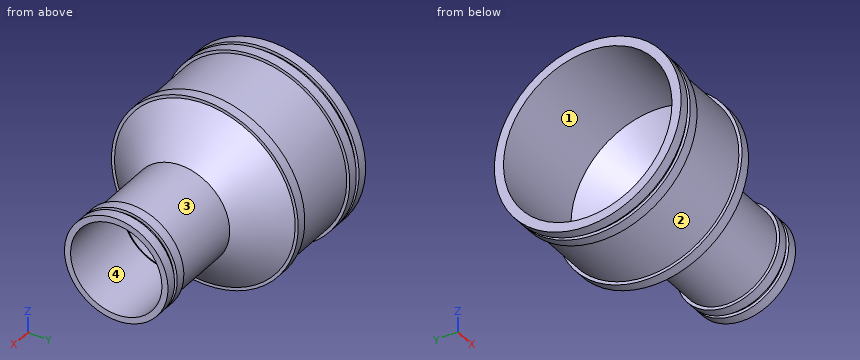
```python
from build123d import *

# Parameters (mm, degrees)
SKELETON_R          = 44.5
SKELETON_R_2        = 41.5
BOSS_EXTRUDE1_DEPTH = 51
BOSS_EXTRUDE2_START = 69
SKELETON_3_R        = 24
SKELETON_3_R_2      = 22
BOSS_EXTRUDE2_DEPTH = 49
SKETCH4_W           = 5
SKETCH4_H           = 1.5
SKETCH6_R           = 22.5
CUT_EXTRUDE1_DEPTH  = 39


with BuildPart() as part:
    # Skeleton → Boss-Extrude1 (new body)
    with BuildSketch(Plane(origin=(0, 0, 0), x_dir=(0, 0, -1), z_dir=(1, 0, 0))):
        Circle(SKELETON_R)
        Circle(SKELETON_R_2, mode=Mode.SUBTRACT)
    extrude(amount=BOSS_EXTRUDE1_DEPTH)



with BuildPart() as body_2:
    # Skeleton<3> → Boss-Extrude2 (new body)
    with BuildSketch(Plane(origin=(0, 0, 0), x_dir=(0, 0, -1), z_dir=(1, 0, 0)).offset(BOSS_EXTRUDE2_START)):
        Circle(SKELETON_3_R)
        Circle(SKELETON_3_R_2, mode=Mode.SUBTRACT)
    extrude(amount=BOSS_EXTRUDE2_DEPTH)


with BuildPart() as part_1:
    add(part.part)

    add(body_2.part)  # loft1 joins it to this body
    # loft up to a face of the part (loft1)
    loft([Face(Wire([part_1.edges().sort_by_distance((51, 32.43910392, 30.462346214))[0]])), Face(Wire([part_1.edges().sort_by_distance((69, -17.495247058, 16.429130542))[0]]))])

    # Cut-Loft1: read off the stored shape, not the designer's step
    # Cut-Loft1: loft between two sections, ruled curve by curve
    cut_loft1_from = [
        Edge.make_bspline([(69, 9.116262782, -20.022331355), (69, -30.928399928, -38.254856919), (69, -49.160925492, 1.789805791), (69, -9.116262782, 20.022331355), (69, 30.928399928, 38.254856919), (69, 49.160925492, -1.789805791), (69, 9.116262782, -20.022331355)], [0, 0, 0, 0, 0.5, 0.5, 0.5, 1, 1, 1, 1], 3, [1, 0.333333333, 0.333333333, 1, 0.333333333, 0.333333333, 1]),
    ]
    cut_loft1_to = [
        Edge.make_bspline([(51, 27.366118575, -31.198486408), (51, -35.030854242, -85.930723557), (51, -89.763091391, -23.533750741), (51, -27.366118575, 31.198486408), (51, 35.030854242, 85.930723557), (51, 89.763091391, 23.533750741), (51, 27.366118575, -31.198486408)], [0, 0, 0, 0, 0.5, 0.5, 0.5, 1, 1, 1, 1], 3, [1, 0.333333333, 0.333333333, 1, 0.333333333, 0.333333333, 1]),
    ]
    cut_loft1 = Solid(Shell([*[Face.make_surface_from_curves(cut_loft1_from[k], cut_loft1_to[k]) for k in range(1)], Face(Wire(cut_loft1_from)), Face(Wire(cut_loft1_to))]))
    add(cut_loft1, mode=Mode.SUBTRACT)

    # Sketch4 → Revolve1 (revolve)
    with BuildSketch(Plane.XY, mode=Mode.PRIVATE) as revolve1_sk:
        with Locations((9.5, 45.25)):
            Rectangle(SKETCH4_W, SKETCH4_H)
        with Locations((2.5, 45.25)):
            Rectangle(SKETCH4_W, SKETCH4_H)
        with Locations((48.5, 45.25)):
            Rectangle(SKETCH4_W, SKETCH4_H)
        with Locations((108.5, 24.75)):
            Rectangle(SKETCH4_W, SKETCH4_H)
        with Locations((115.5, 24.75)):
            Rectangle(SKETCH4_W, SKETCH4_H)
    revolve(revolve1_sk.sketch.rotate(Axis((0, 0, 0), (1, 0, 0)), 90), axis=Axis((0, 0, 0), (1, 0, 0)))

    # Sketch6 → Cut-Extrude1 (cut)
    with BuildSketch(Plane(origin=(118, 0, 0), x_dir=(0, 0, -1), z_dir=(1, 0, 0))):
        Circle(SKETCH6_R)
    extrude(amount=-CUT_EXTRUDE1_DEPTH, mode=Mode.SUBTRACT)


solid = part_1.part
```
Geometry check sheet. Reference: the model listing, model coordinates, mm. Face numbers are marked on the shaded views. A direction names the side the tool comes from. Coordinates: 2 decimals unless noted, no trailing zeros. Loops run counter-clockwise (first coordinate to the right, second up) from the corner with the lowest first, then second, coordinate; pieces in that order, holes last.
Item 1: Sectioned sample at A-A, the plane x = 91. Record the boundary of the cut face in (y, z).
Item 2: Go/stop test with flat-tipped pins: pin 1 Ø8 at (y, z) = (-28.5, 13.5) entering from -X; pin 2 Ø10 at (x, y) = (72.5, -19) entering from -Z; pin 3 Ø10 at (x, y) = (60, -34) entering from +Z; pin 4 Ø10 at (y, z) = (15, -23.5) entering from +X. Record where each tip stops, or that it passes through.
Item 3: Release check for a two-part mould opening along Y. For the marked faces 1 and 2 record: released by +Y, released by -Y, zero draft, split by the parting line, or undercut.
Item 4: Access from +Z, -Z, +X, -X, +Y, -Y to the whole of each face (thin tool, end or side, straight path). Record for the marked faces 3 and 4.
Item 5: Thickness scan on line 1 (X direction, y = 31.5, z = -32.5); line 2 (Z direction, x = 76, y = 0); line 3 (Y direction, x = 16, z = 0). Record the ranges inside material, lowest first.
Check result:
1. outline: circle Ø48 at (0, 0); hole circle Ø45 at (0, 0)
2. pin 1: stops at x = 56.3
2. pin 2: stops at z = -19.49
2. pin 3: stops at z = 23.35
2. pin 4: stops at x = 118
3. face 1: undercut
3. face 2: split by the parting line
4. face 3: none
4. face 4: +X
5. line 1: x = 0 to 5, 7 to 12, 46 to 51
5. line 2: z = -24 to -22, 22 to 24
5. line 3: y = -44.5 to -41.5, 41.5 to 44.5
